Check sheet for the modelled part. Datum: model origin and axes. Units: mm. Face numbers are marked on the shaded views. Round coordinates to 2 decimals unless told otherwise and drop trailing zeros. Loops run counter-clockwise (first coordinate to the right, second up) from the corner with the lowest first, then second, coordinate; pieces in that order, holes last. Notation, with made-up numbers: (39.25, 46) - (50.25, 46) arc R16 ccw to (50.25, 60) - close; hole circle Ø7 at (-14, 27). An arc over 180 degrees is marked (long way). Return JSON: item names as keys, results as strings.
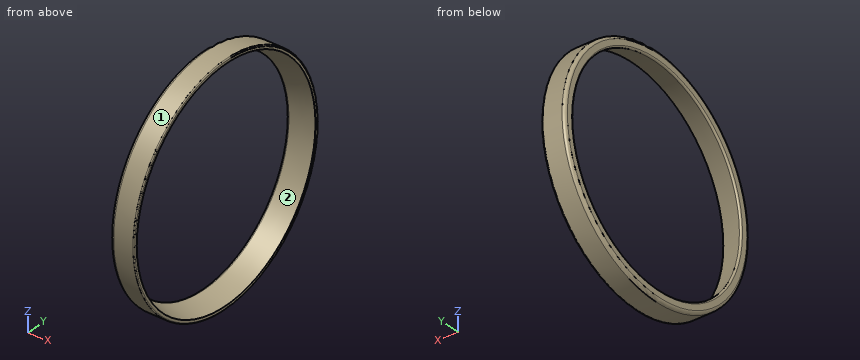
Autodesk Inventor part; units mm, degrees
ref_plane "outer_ring_XY" through (0, 0, 0) normal (0, 0, 1) x (1, 0, 0)
ref_plane "outer_ring_YZ" through (0, 0, 0) normal (1, 0, 0) x (0, 1, 0)
ref_plane "outer_ring_ZX" through (0, 0, 0) normal (0, 1, 0) x (0, 0, 1)
sketch "Sketch_1" plane through (0, 0, 0) normal (0, 0, 1) x (1, 0, 0)
  line L0 (23, 0) -> (-23, 0)
  arc A0 (0, 106.4915) -> (1.9411, 105.0578) centre (1.5, 106.4915) ccw
  line L1 (1.9411, 105.0578) -> (23, 111.5364)
  line L2 (23, 111.5364) -> (23, 114)
  arc A1 (23, 114) -> (22, 115) centre (22, 114) ccw
  line L3 (22, 115) -> (3, 115)
  arc A2 (3, 115) -> (0, 112) centre (3, 112) ccw
  line L4 (0, 112) -> (0, 106.4915)
revolve "Revolution1" add sketch "Sketch_1" angle 360 about axis through (23, 0, 0) along (1, 0, 0)
ref_plane "outer_ring_XY" through (0, 0, 0) normal (0, 0, 1) x (1, 0, 0)
ref_plane "outer_ring_YZ" through (0, 0, 0) normal (1, 0, 0) x (0, 1, 0)
ref_plane "outer_ring_ZX" through (0, 0, 0) normal (0, 1, 0) x (0, 0, 1)
properties part number "T4DB 170_or"
Q1. Draft check along Z on the marked faces 1 and 2. Enter one of: released by +Z, released by -Z, zero draft, split by the parting line, or undercut.
Answer key:
{"face 1": "split by the parting line", "face 2": "undercut"}
Q2. Sectioned sample at A-A (z = 0). Enter the section's corners in (x, y), plus the area to 3 significant figures.
Answer key:
{"outline": "(0, -112) arc R3 ccw to (3, -115) - (22, -115) arc R1 ccw to (23, -114) - (23, -111.54) - (1.94, -105.06) arc R1.5 ccw to (0, -106.49) - close; (0, 106.49) arc R1.5 ccw to (1.94, 105.06) - (23, 111.54) - (23, 114) arc R1 ccw to (22, 115) - (3, 115) arc R3 ccw to (0, 112) - close", "area": "316 mm²"}
Q3. Depth check by flat-ended pin: P1, Ø1, axis at x = 10, z = 54.5, coming from the -Y side; P2, Ø10, axis at x = 20.5, y = 16.5, coming from the +Z side; P3, Ø4, axis at x = 5.5, y = -10.5, coming from the -Z side. Enter the tip coordinate at first touch or a pass-through.
Answer key:
{"P1": "stops at y = -101.53", "P2": "stops at z = 114.42", "P3": "stops at z = -114.69"}
Q4. Sectioned sample at C-C (x = 11). Enter the section's corners in (y, z), plus the area to 3 significant figures.
Answer key:
{"outline": "circle Ø230 at (0, 0); hole circle Ø215.69 at (0, 0)", "area": "5,010 mm²"}
Q5. Scan lines: probe 1 along Y at (x, z) = (12.5, 5.5); probe 2 along Z at (x, y) = (9.25, -9.5); probe 3 along Y at (x, z) = (12.75, -32.5). Record each from-to range of solid material in increasing order. Write a range as [from, to].
Answer key:
{"probe 1": "y = [-114.87, -108.17], [108.17, 114.87]", "probe 2": "z = [-114.61, -106.88], [106.88, 114.61]", "probe 3": "y = [-110.31, -103.4], [103.4, 110.31]"}
